Design review of the part built by this model. Coordinates are the model's own, in mm. Face numbers are marked on the shaded views. A direction names the side the tool comes from. Round coordinates to 2 decimals unless told otherwise and drop trailing zeros. Loops run counter-clockwise (first coordinate to the right, second up) from the corner with the lowest first, then second, coordinate; pieces in that order, holes last. Notation, with made-up numbers: (16, 31) - (29, 31) arc R21 ccw to (29, 55) - close; hole circle Ø10 at (-35, -24.75). An arc over 180 degrees is marked (long way). Answer as CSV lines item,"result". Start each with the question number.
(1) For the marked faces 1 and 2, list the 3-axis set-ups (+Z, -Z, +X, -X, +Y, -Y) from which the entire face can be reached by the end or side of a thin tool; tool diameter is ignored.
(2) Wall thickness on L1, parallel to Z at x = 0, y = -2; L2, parallel to Y at x = -0.5, z = 3.25; L3, parallel to X at y = -1, z = 0.25: over which ranges is each line inside the solid? List them lowest first.
(3) Mouldability with a two-part tool opening along Z and no side actions: class the marked faces 3, 4 and 5 as released by +Z, released by -Z, zero draft, split by the parting line, or undercut.
(4) For P1, Ø3, axis at x = -4.5, y = 1, coming from the +Z side; P2, Ø2, axis at x = -3, y = 1.5, coming from the -Z side; P3, Ø0.7, axis at y = 2, z = 1, coming from the +X side, all flat-tipped, find the tip position at first contact; note any pin that passes through.
(5) Consider section D-D (z = 3). Give the boundary of the cut face in (x, y), and give its area (3 significant figures).
(6) Consider section C-C (y = -2.5). Give the boundary of the cut face in (x, z), and give its area (3 significant figures).
(7) Consider section B-B (x = -5). Give the boundary of the cut face in (y, z).
(8) Consider section A-A (x = -1.25). Give the boundary of the cut face in (y, z), and give its area (3 significant figures).
from build123d import *

# Parameters (mm, degrees)
SKETCH1_W       = 3
SKETCH1_H       = 2.5
EXTRUDE1_DEPTH  = 5
SKETCH2_W       = 0.645
SKETCH2_H       = 3.5
EXTRUDE2_DEPTH  = 0.64
LPATTERN1_COUNT = 4
LPATTERN1_PITCH = 2.54
CHAMFER1_SIZE   = 0.25


with BuildPart() as part:
    # Sketch1 → Extrude1 (new body, symmetric)
    with BuildSketch(Plane.XY):
        Rectangle(SKETCH1_W, SKETCH1_H)
    extrude(amount=EXTRUDE1_DEPTH, both=True)

    # Sketch2 → Extrude2 (add)
    with BuildSketch(Plane.XY.offset(3.86)):
        with BuildLine():
            Line((-0.3225, 1.25), (-0.3225, 2.245))
            ThreePointArc((-0.3225, 2.245), (-0.374776878, 2.375), (-0.5025, 2.43261663))
            Line((-0.5025, 2.43261663), (-6.5025, 2.43261663))
            Line((-6.5025, 2.43261663), (-6.5025, 3.06831282))
            Line((-6.5025, 3.06831282), (-0.4975, 3.06831282))
            ThreePointArc((-0.4975, 3.06831282), (0.082527742, 2.826), (0.3225, 2.245))
            Line((0.3225, 2.245), (0.3225, 1.25))
            Line((0.3225, 1.25), (-0.3225, 1.25))
        make_face()
        with Locations((0, -3)):
            Rectangle(SKETCH2_W, SKETCH2_H)
    extrude2 = extrude(amount=-EXTRUDE2_DEPTH)

    # LPattern1: Extrude2 ×4
    with Locations(*[(0, 0, -i * LPATTERN1_PITCH) for i in range(1, LPATTERN1_COUNT)]):
        add(extrude2)

    # Chamfer1
    chamfer1_edges = [part.edges().sort_by_distance(p)[0] for p in [
        (-6.5025, 2.750464725, -4.4),
        (-6.5025, 2.43261663, -4.08),
        (-6.5025, 3.06831282, -4.08),
        (-6.5025, 2.750464725, -3.76),
        (0, -4.75, -4.4),
        (0.3225, -4.75, -4.08),
        (-0.3225, -4.75, -4.08),
        (0, -4.75, -3.76),
        (-6.5025, 2.750464725, 3.22),
        (-6.5025, 2.43261663, 3.54),
        (-6.5025, 3.06831282, 3.54),
        (-6.5025, 2.750464725, 3.86),
        (0, -4.75, 3.22),
        (0.3225, -4.75, 3.54),
        (-0.3225, -4.75, 3.54),
        (0, -4.75, 3.86),
        (-6.5025, 2.750464725, 0.68),
        (-6.5025, 2.43261663, 1),
        (-6.5025, 3.06831282, 1),
        (-6.5025, 2.750464725, 1.32),
        (0, -4.75, 0.68),
        (0.3225, -4.75, 1),
        (-0.3225, -4.75, 1),
        (0, -4.75, 1.32),
        (-6.5025, 2.750464725, -1.86),
        (-6.5025, 2.43261663, -1.54),
        (-6.5025, 3.06831282, -1.54),
        (-6.5025, 2.750464725, -1.22),
        (0, -4.75, -1.86),
        (0.3225, -4.75, -1.54),
        (-0.3225, -4.75, -1.54),
        (0, -4.75, -1.22),
    ]]
    chamfer(chamfer1_edges, length=CHAMFER1_SIZE)


solid = part.part
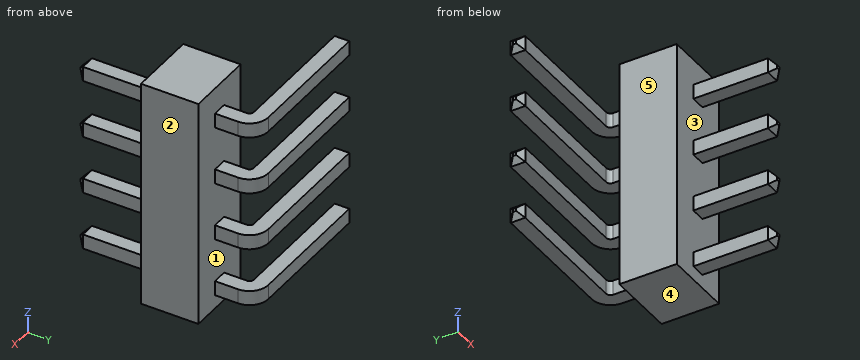
Determined:
1,face 1,"none"
1,face 2,"+Z, -Z, +X, +Y, -Y"
2,L1,"z = -4.4 to -3.76, -1.86 to -1.22, 0.68 to 1.32, 3.22 to 3.86"
2,L2,"y = -1.25 to 1.25, 2.43 to 3.07"
2,L3,"x = -1.5 to 1.5"
3,face 3,"undercut"
3,face 4,"released by -Z"
3,face 5,"zero draft"
4,P1,"stops at z = 3.86"
4,P2,"stops at z = -4.4"
4,P3,"stops at x = 0.32"
5,outline,"(-1.5, -1.25) - (1.5, -1.25) - (1.5, 1.25) - (-1.5, 1.25) - close"
5,area,"7.50 mm^2"
6,outline,"(-0.32, -4.4) - (0.32, -4.4) - (0.32, -3.76) - (-0.32, -3.76) - close; (-0.32, -1.86) - (0.32, -1.86) - (0.32, -1.22) - (-0.32, -1.22) - close; (-0.32, 0.68) - (0.32, 0.68) - (0.32, 1.32) - (-0.32, 1.32) - close; (-0.32, 3.22) - (0.32, 3.22) - (0.32, 3.86) - (-0.32, 3.86) - close"
6,area,"1.65 mm^2"
7,outline,"(2.43, -4.4) - (3.07, -4.4) - (3.07, -3.76) - (2.43, -3.76) - close; (2.43, -1.86) - (3.07, -1.86) - (3.07, -1.22) - (2.43, -1.22) - close; (2.43, 0.68) - (3.07, 0.68) - (3.07, 1.32) - (2.43, 1.32) - close; (2.43, 3.22) - (3.07, 3.22) - (3.07, 3.86) - (2.43, 3.86) - close"
8,outline,"(-1.25, -5) - (1.25, -5) - (1.25, 5) - (-1.25, 5) - close; (2.43, -4.4) - (3.07, -4.4) - (3.07, -3.76) - (2.43, -3.76) - close; (2.43, -1.86) - (3.07, -1.86) - (3.07, -1.22) - (2.43, -1.22) - close; (2.43, 0.68) - (3.07, 0.68) - (3.07, 1.32) - (2.43, 1.32) - close; (2.43, 3.22) - (3.07, 3.22) - (3.07, 3.86) - (2.43, 3.86) - close"
8,area,"26.6 mm^2"
